Input: part model. Units: mm. Frame: model coordinates. A direction names the side the tool comes from. Round coordinates to 2 decimals unless told otherwise and drop trailing zeros. Order: outer loops, then holes, each group sorted by start corner. A loop starts at its lowest first (then second) coordinate and runs counter-clockwise, first axis right, second up. Notation, with made-up numbers: (5, 16) -> (9, 16) arc R8 cw to (9, 20) -> close; hole circle Ø9 at (28, 21.5). An arc over 180 degrees is marked (long way). Use a Markdown table: item, result.
from build123d import *

# Parameters (mm, degrees)
ESQUISSE1_W                               = 256
ESQUISSE1_H                               = 100
T_LE_DE_BASE_PLI_E1_DEPTH                 = 10
ENL_V_MAT_EXTRU_1_DEPTH                   = 10
TROU_POUR_TARAUDAGE_POUR_TROU_TARAUD_M1_D = 14
TAB_START                                 = -10
TAB_AND_SLOT_TAB1_DEPTH                   = 10
TAB_AND_SLOT_TAB2_DEPTH                   = 10
TAB_AND_SLOT_TAB3_DEPTH                   = 10
ESQUISSE17_W                              = 256
ESQUISSE17_H                              = 10
ENL_V_MAT_EXTRU_2_DEPTH                   = 10
DIAM_TRE_DU_PER_AGE_2_0_2_1_D             = 2


# Read off the part's stored shape, not the designer's step: Tab and Slot-Tab1, Tab and Slot-Tab2, Tab and Slot-Tab3
# Sheet-metal steps are written as plain solids
with BuildPart() as part:
    # Esquisse1 → Tôle de base pliée1 (new body)
    with BuildSketch(Plane.XY):
        with Locations((128, 50)):
            Rectangle(ESQUISSE1_W, ESQUISSE1_H)
    extrude(amount=-T_LE_DE_BASE_PLI_E1_DEPTH)

    # Esquisse9 → Enlèv. mat.-Extru.1 (cut)
    with BuildSketch(Plane.XY):
        with BuildLine():
            Line((32, 100), (110, 100))
            ThreePointArc((110, 100), (71, 139), (32, 100))
        make_face()
        with BuildLine():
            ThreePointArc((32, 100), (71, 61), (110, 100))
            Line((110, 100), (32, 100))
        make_face()
        with BuildLine():
            ThreePointArc((224, 100), (185, 139), (146, 100))
            Line((146, 100), (224, 100))
        make_face()
        with BuildLine():
            Line((224, 100), (146, 100))
            ThreePointArc((146, 100), (185, 61), (224, 100))
        make_face()
    extrude(amount=-ENL_V_MAT_EXTRU_1_DEPTH, mode=Mode.SUBTRACT)

    # Trou pour taraudage pour trou taraudé M161 (through all)
    with Locations(Plane.XY):
        with Locations((71, 26), (185, 26)):
            Hole(TROU_POUR_TARAUDAGE_POUR_TROU_TARAUD_M1_D / 2)

    # Tab and Slot-Tab1 outline → Tab and Slot-Tab1 (add)
    with BuildSketch(Plane.XY.offset(TAB_START)):
        Polygon((204, -10), (206, -8), (206, 0), (166, 0), (166, -8), (168, -10), align=None)
        Polygon((90, -8), (90, 0), (50, 0), (50, -8), (52, -10), (88, -10), align=None)
    extrude(amount=TAB_AND_SLOT_TAB1_DEPTH)

    # Tab and Slot-Tab2 outline → Tab and Slot-Tab2 (add)
    with BuildSketch(Plane.XY.offset(TAB_START)):
        Polygon((-10, 17), (-8, 15), (0, 15), (0, 40), (-8, 40), (-10, 38), align=None)
        Polygon((-8, 65), (0, 65), (0, 90), (-8, 90), (-10, 88), (-10, 67), align=None)
    extrude(amount=TAB_AND_SLOT_TAB2_DEPTH)

    # Tab and Slot-Tab3 outline → Tab and Slot-Tab3 (add)
    with BuildSketch(Plane.XY.offset(TAB_START)):
        Polygon((256, 90), (256, 65), (264, 65), (266, 67), (266, 88), (264, 90), align=None)
        Polygon((256, 15), (264, 15), (266, 17), (266, 38), (264, 40), (256, 40), align=None)
    extrude(amount=TAB_AND_SLOT_TAB3_DEPTH)

    # Esquisse17 → Enlèv. mat.-Extru.2 (cut)
    with BuildSketch(Plane.XY):
        with Locations((128, 95)):
            Rectangle(ESQUISSE17_W, ESQUISSE17_H)
    extrude(amount=-ENL_V_MAT_EXTRU_2_DEPTH, mode=Mode.SUBTRACT)

    # Diamètre du perçage Ø2.0 (2)1 (through all)
    with Locations(Plane.XY):
        with Locations((256, 64)):
            diam_tre_du_per_age_2_0_2_1 = Hole(DIAM_TRE_DU_PER_AGE_2_0_2_1_D / 2)

    # Répét. par esquisse1: Diamètre du perçage Ø2.0 (2)1 at 9 more places
    with Locations((-256, 0, 0), (-256, -23, 0), (-256, -50, 0), (-207, -64, 0), (-165, -64, 0), (-91, -64, 0), (-49, -64, 0), (0, -50, 0), (0, -23, 0)):
        add(diam_tre_du_per_age_2_0_2_1, mode=Mode.SUBTRACT)


solid = part.part
1) Pin query (flat end, axial travel): pin 1 Ø22.5 at (x, y) = (71, 26) entering from +Z; pin 2 Ø5 at (x, z) = (242, -6.5) entering from -Y; pin 3 Ø2.5 at (y, z) = (-2.5, -6.5) entering from +X; pin 4 Ø3 at (y, z) = (4, -4) entering from -X. Return the tip coordinate at first contact, or that it passes through.
Results found:
| item | result |
|---|---|
| pin 1 | stops at z = 0 |
| pin 2 | stops at y = 0 |
| pin 3 | stops at x = 206 |
| pin 4 | stops at x = 0 |
2) Set-up query: faces 1 (the flat face through (-4, 65, -5)), 2 (the flat face through (256, 6, -5)), 3 (the flat face through (166, -4, -5)). Return all of +Z, -Z, +X, -X, +Y, -Y with unobstructed straight access to the full face (end or side cutting, diameter ignored); none if empty.
Results found:
| item | result |
|---|---|
| face 1 | +Z, -Z, -X |
| face 2 | +Z, -Z, +X, -Y |
| face 3 | +Z, -Z, -Y |
3) Cut plane A-A on x = 185. Return loops of the section in (y, z).
Results found:
| item | result |
|---|---|
| outline | (-10, -10) -> (19, -10) -> (19, 0) -> (-10, 0) -> close; (33, -10) -> (61, -10) -> (61, 0) -> (33, 0) -> close |
4) Cut plane C-C on z = -3. Count the separate pieces of the cut face and the enclosed holes in it, and give its area (3 significant figures).
Results found:
| item | result |
|---|---|
| separate pieces | 1 |
| enclosed holes | 2 |
| area | 21,300 mm² |
5) Cut plane D-D on y = 7. Return loops of the section in (x, z).
Results found:
| item | result |
|---|---|
| outline | (0, -10) -> (256, -10) -> (256, 0) -> (0, 0) -> close |
6) Cut plane B-B on y = 76. Return loops of the section in (x, z), and give its area (3 significant figures).
Results found:
| item | result |
|---|---|
| outline | (-10, -10) -> (40.26, -10) -> (40.26, 0) -> (-10, 0) -> close; (101.74, -10) -> (154.26, -10) -> (154.26, 0) -> (101.74, 0) -> close; (215.74, -10) -> (266, -10) -> (266, 0) -> (215.74, 0) -> close |
| area | 1,530 mm² |
7) Line query: L1, parallel to X at y = -2, z = -2; L2, parallel to X at y = 84.5, z = -7; L3, parallel to X at y = 1.5, z = -5.5. Output: solid intervals per line, ascending. Write a range as [from, to].
Results found:
| item | result |
|---|---|
| L1 | x = [50, 90], [166, 206] |
| L2 | x = [-10, 35.21], [106.79, 149.21], [220.79, 266] |
| L3 | x = [0, 256] |
